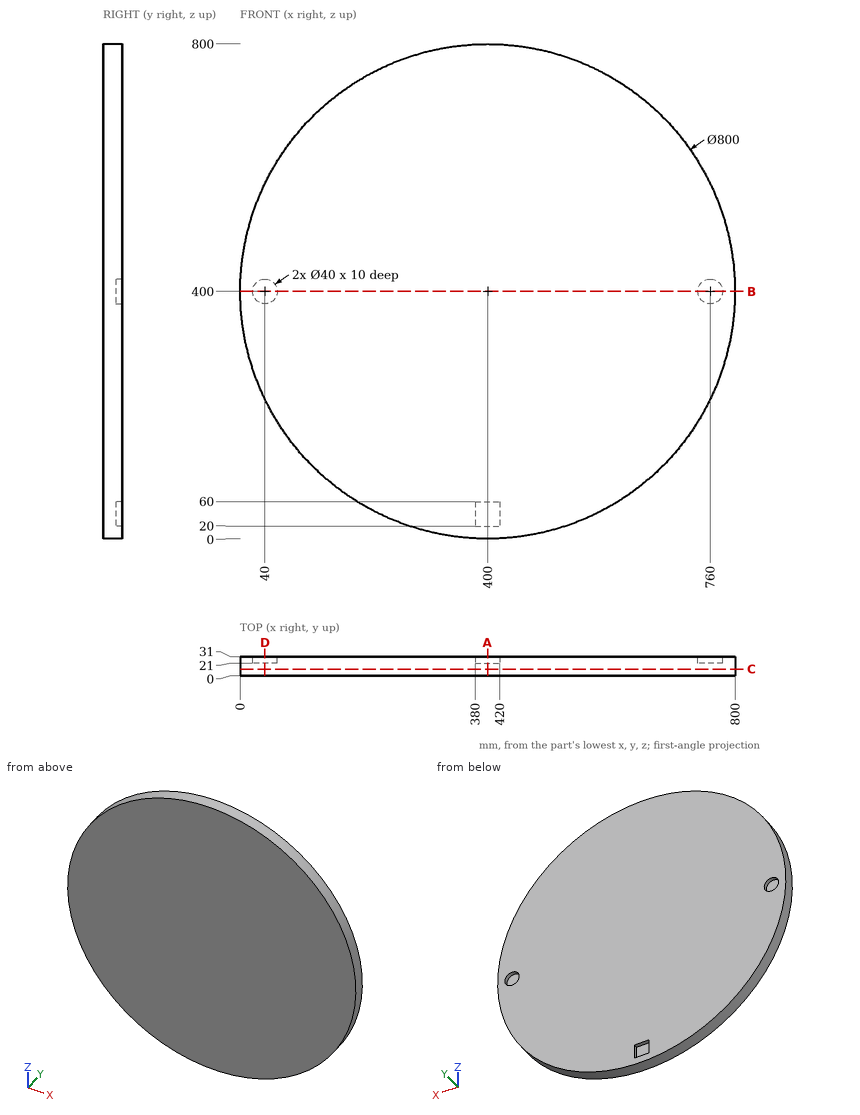
The figure shows three views and two pictorial views of one solid part (mm, origin at its lowest corner). Answer the questions. Coordinates: 2 decimals unless noted, no trailing zeros. Loops run counter-clockwise (first coordinate to the right, second up) from the corner with the lowest first, then second, coordinate; pieces in that order, holes last. Notation, with made-up numbers: (20.25, 53.5) - (77.25, 53.5) arc R29 ccw to (77.25, 79.5) - close; hole circle Ø2 at (-20.5, 67). An arc over 180 degrees is marked (long way). Answer in a Markdown table with one row per item.
Q1. Given P1, Ø20, axis at x = 751, z = 396.5, coming from the +Y side; P2, Ø11, axis at y = 27.5, z = 48.5, coming from the -X side; P3, Ø5, axis at x = 403, y = 27.5, coming from the +Z side; P4, Ø10, axis at x = 344.5, z = 112, coming from the -Y side, each flat-ended and moving along its own axis, determine where each tip first touches the part or whether it passes through.
Here are the results:
| item | result |
|---|---|
| P1 | stops at y = 21 |
| P2 | stops at x = 199.29 |
| P3 | stops at z = 800 |
| P4 | stops at y = 0 |
Q2. Straight lines are drawn through the part: line 1 along X through (y, z) = (25.5, 400); line 2 along X through (y, z) = (24, 382.5); line 3 along Z through (x, y) = (718, 3). For each, find the intervals that lie inside material, in ascending order. Write a range as [from, to].
Here are the results:
| item | result |
|---|---|
| line 1 | x = [0, 20], [60, 740], [780, 800] |
| line 2 | x = [0.38, 30.32], [49.68, 750.32], [769.68, 799.62] |
| line 3 | z = [157.36, 642.64] |
Q3. Find section D-D on x = 40. Write down the section's boundary in (y, z), plus the area to 3 significant figures.
Here are the results:
| item | result |
|---|---|
| outline | (0, 225.64) - (31, 225.64) - (31, 380) - (21, 380) - (21, 420) - (31, 420) - (31, 574.36) - (0, 574.36) - close |
| area | 10,400 mm^2 |
Q4. Find section B-B on z = 400. Write down the section's boundary in (x, y).
Here are the results:
| item | result |
|---|---|
| outline | (0, 0) - (800, 0) - (800, 31) - (780, 31) - (780, 21) - (740, 21) - (740, 31) - (60, 31) - (60, 21) - (20, 21) - (20, 31) - (0, 31) - close |
Q5. Find section A-A on x = 400. Write down the section's boundary in (y, z).
Here are the results:
| item | result |
|---|---|
| outline | (0, 0) - (31, 0) - (31, 20) - (21, 20) - (21, 60) - (31, 60) - (31, 800) - (0, 800) - close |
Q6. Find section C-C on y = 11. Write down the section's boundary in (x, z).
Here are the results:
| item | result |
|---|---|
| outline | circle Ø800 at (400, 400) |
